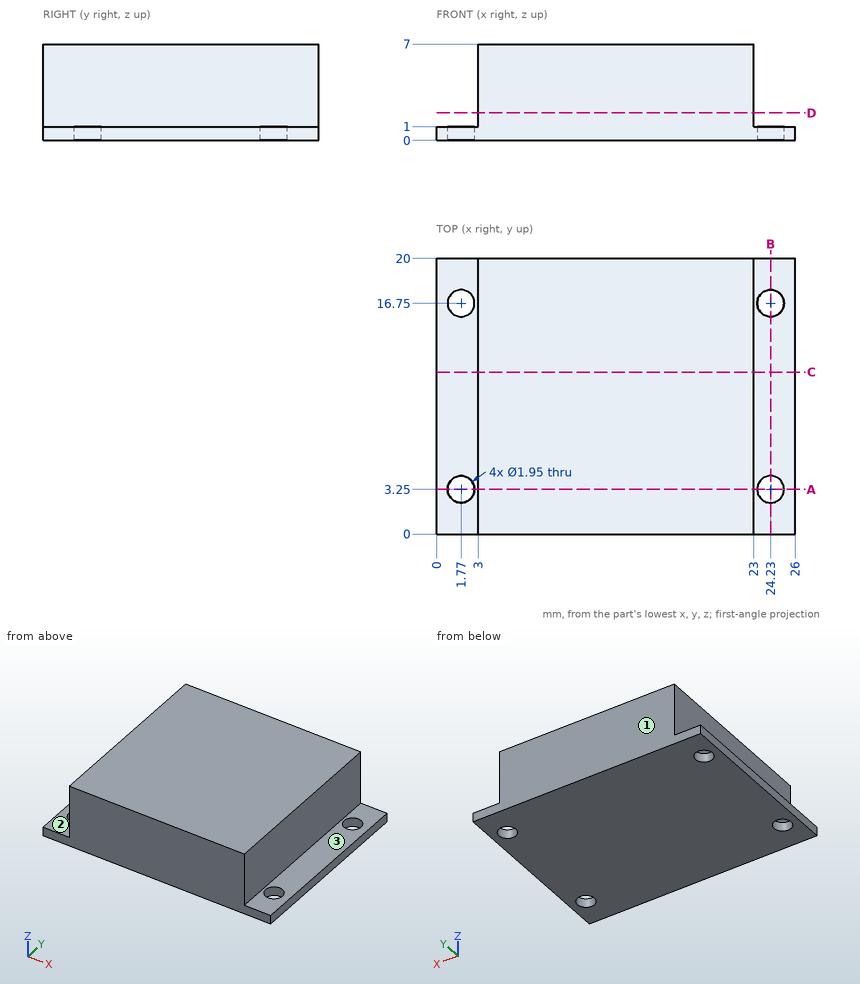
The drawing under review shows one solid part. Ordinate dimensions are in mm from its lowest x, y, z. A direction names the side the tool comes from. Round coordinates to 2 decimals unless told otherwise and drop trailing zeros. Loops run counter-clockwise (first coordinate to the right, second up) from the corner with the lowest first, then second, coordinate; pieces in that order, holes last. Notation, with made-up numbers: (10.5, -37) -> (33.5, -37) arc R20 ccw to (33.5, -2) -> close; hole circle Ø5 at (5, 85). An arc over 180 degrees is marked (long way). Answer in a Markdown table with one row per item.
1) Wall thickness on line 1 along Y through (x, z) = (24.23, 0.6) (3 decimals); line 2 along X through (y, z) = (3.25, 0.65) (3 decimals); line 3 along X through (y, z) = (12, 4.5): over which ranges is each line inside the solid? List them lowest first.
Taken from the geometry:
| item | result |
|---|---|
| line 1 | y = 0 to 2.275, 4.225 to 15.775, 17.725 to 20 |
| line 2 | x = 0 to 0.795, 2.745 to 23.255, 25.205 to 26 |
| line 3 | x = 3 to 23 |
2) Consider section C-C, the plane y = 11.75. Write out the cut boundary in (x, z), plus the area to 3 significant figures.
Taken from the geometry:
| item | result |
|---|---|
| outline | (0, 0) -> (26, 0) -> (26, 1) -> (23, 1) -> (23, 7) -> (3, 7) -> (3, 1) -> (0, 1) -> close |
| area | 146 mm² |
3) For pin 1 Ø3 at (x, y) = (6.5, 18) entering from -Z; pin 2 Ø1.5 at (x, y) = (1.5, 9) entering from +Z; pin 3 Ø3 at (y, z) = (14.5, 4.5) entering from +X; pin 4 Ø1.6 at (x, y) = (24.23, 16.75) entering from +Z, all flat-tipped, find the tip position at first contact; note any pin that passes through.
Taken from the geometry:
| item | result |
|---|---|
| pin 1 | stops at z = 0 |
| pin 2 | stops at z = 1 |
| pin 3 | stops at x = 23 |
| pin 4 | passes through |
4) Consider section B-B, the plane x = 24.23. Write out the cut boundary in (y, z) (3 decimals).
Taken from the geometry:
| item | result |
|---|---|
| outline | (0, 0) -> (2.275, 0) -> (2.275, 1) -> (0, 1) -> close; (4.225, 0) -> (15.775, 0) -> (15.775, 1) -> (4.225, 1) -> close; (17.725, 0) -> (20, 0) -> (20, 1) -> (17.725, 1) -> close |
5) Consider section A-A, the plane y = 3.25. Write out the cut boundary in (x, z) (3 decimals), plus the area to 3 significant figures.
Taken from the geometry:
| item | result |
|---|---|
| outline | (0, 0) -> (0.795, 0) -> (0.795, 1) -> (0, 1) -> close; (2.745, 0) -> (23.255, 0) -> (23.255, 1) -> (23, 1) -> (23, 7) -> (3, 7) -> (3, 1) -> (2.745, 1) -> close; (25.205, 0) -> (26, 0) -> (26, 1) -> (25.205, 1) -> close |
| area | 142 mm² |
6) Consider section D-D, the plane z = 2. Write out the cut boundary in (x, y).
Taken from the geometry:
| item | result |
|---|---|
| outline | (3, 0) -> (23, 0) -> (23, 20) -> (3, 20) -> close |
7) Tool access review of the marked faces 1, 2 and 3: name each direction out of +Z, -Z, +X, -X, +Y, -Y from which nothing blocks a thin tool from reaching the whole face with its end or side.
Taken from the geometry:
| item | result |
|---|---|
| face 1 | +Z, -Z, +X, -X, +Y |
| face 2 | +Z, -X, +Y, -Y |
| face 3 | +Z, +X, +Y, -Y |
